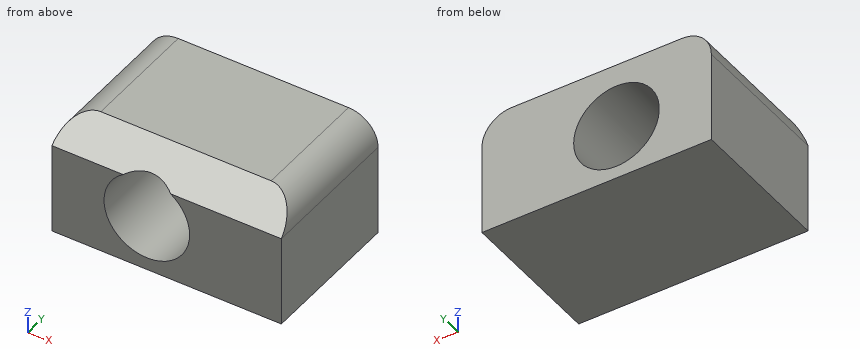
```python
from build123d import *

# Parameters (mm, degrees)
F0_W        = 39.4569858909
F0_H        = 20.7027406432
F1_DEPTH    = 25.4
F2_R        = 7.3634612469
F3_DEPTH    = 25.4
F4_T1_DEPTH = 65.5852850486
F5_R        = 5.08
F6_R        = 5.08


# Not quite as in the source:
# - a fillet or chamfer that OpenCascade refuses, or shapes differently, is made with other operations: its cross-section is extruded or revolved along the edge and cut away or added


with BuildPart() as f1:
    # F0 (on Front) → F1 (new body)
    with BuildSketch(Plane.XZ):
        with Locations((-6.9415066391, 7.18506868)):
            Rectangle(F0_W, F0_H)
    extrude(amount=F1_DEPTH)

    # F2 (on face) → F3 (cut)
    with BuildSketch(Plane.XZ.offset(25.4)):
        with Locations((-10.3513691574, 6.3326032832)):
            Circle(F2_R)
    extrude(amount=-F3_DEPTH, mode=Mode.SUBTRACT)

    # F4: chamfer of 5.08 on 1 edges, made by hand

    # F4_s2 → F4_t1 (cut)
    with BuildSketch(Plane.YZ.offset(-39.7341491634)):
        Polygon((-20.32, 17.5364390016), (-25.4, 12.4564390016), (-25.4, 17.5364390016), align=None)
    extrude(amount=F4_T1_DEPTH, mode=Mode.SUBTRACT)

    # F5
    f5_edges = [f1.edges().sort_by_distance(p)[0] for p in [
        (12.786986, -10.16, 17.536439),
    ]]
    fillet(f5_edges, radius=F5_R)

    # F6
    f6_edges = [f1.edges().sort_by_distance(p)[0] for p in [
        (-26.67, -10.16, 17.536439),
    ]]
    fillet(f6_edges, radius=F6_R)


solid = f1.part
```
Input: part model. Units: mm. Frame: model coordinates. Round coordinates to 2 decimals unless told otherwise and drop trailing zeros. Loops run counter-clockwise (first coordinate to the right, second up) from the corner with the lowest first, then second, coordinate; pieces in that order, holes last.
1) Section query B-B on x = -13. Return the cut outline in (y, z), plus the area to 3 significant figures.
Ans:
outline: (-25.4, -3.17) - (0, -3.17) - (0, -0.54) - (-25.4, -0.54) - close; (-24.65, 13.2) - (0, 13.2) - (0, 17.54) - (-20.32, 17.54) - close
area: 164 mm2
2) Section query D-D on x = -2. Return the cut outline in (y, z), plus the area to 3 significant figures.
Ans:
outline: (-25.4, -3.17) - (0, -3.17) - (0, 17.54) - (-20.32, 17.54) - (-25.4, 12.46) - close
area: 513 mm2
3) Material intervals for line 1 (X direction, y = -6, z = 6.5); line 2 (X direction, y = -15, z = 0.5); line 3 (Z direction, x = -10.5, y = -17.75), sorted ascending.
Ans:
line 1: x = -26.67 to -17.71, -2.99 to 12.79
line 2: x = -26.67 to -14.85, -5.86 to 12.79
line 3: z = -3.17 to -1.03, 13.69 to 17.54
4) Section query C-C on y = -7.75. Return the cut outline in (x, z).
Ans:
outline: (-26.67, -3.17) - (12.79, -3.17) - (12.79, 12.46) arc R5.08 ccw to (7.71, 17.54) - (-21.59, 17.54) arc R5.08 ccw to (-26.67, 12.46) - close; hole circle Ø14.73 at (-10.35, 6.33)
5) Section query A-A on z = 9. Return the cut outline in (x, y), plus the area to 3 significant figures.
Ans:
outline: (-26.67, -25.4) - (-17.21, -25.4) - (-17.21, 0) - (-26.67, 0) - close; (-3.49, -25.4) - (12.79, -25.4) - (12.79, 0) - (-3.49, 0) - close
area: 654 mm2
